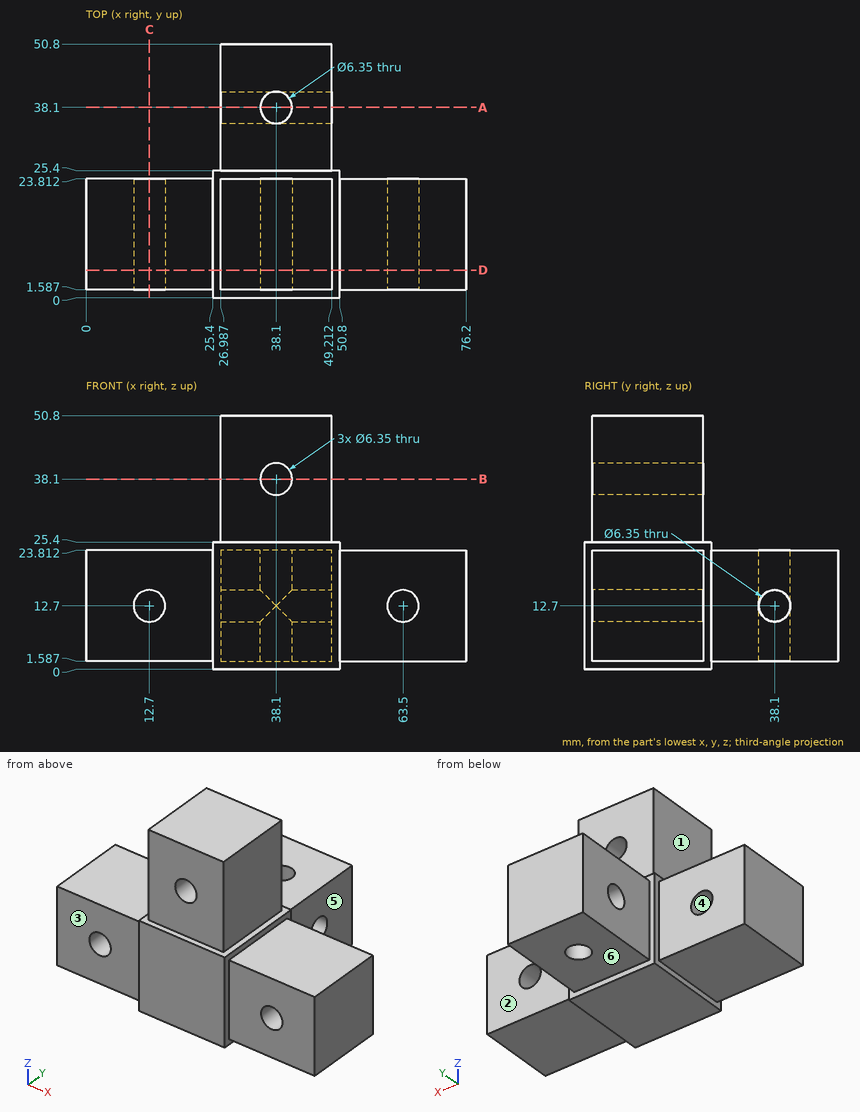
For this review, use the dimensioned drawing (mm, ordinates from the lowest corner) and the shaded views. A direction names the side the tool comes from. Round coordinates to 2 decimals unless told otherwise and drop trailing zeros. Order: outer loops, then holes, each group sorted by start corner. A loop starts at its lowest first (then second) coordinate and runs counter-clockwise, first axis right, second up. Notation, with made-up numbers: M 46.5,58 L 71.5,58 A20 cw 71.5,68 Z; hole C -28,55 d7. An arc over 180 degrees is marked long. Use a Markdown table: item, result.
1) Consider section A-A (y = 38.1). Write out the cut boundary in (x, z) (1 decimal).
Report:
| item | result |
|---|---|
| outline | M 27,1.6 L 34.9,1.6 L 34.9,9.5 L 27,9.5 Z; M 27,15.9 L 34.9,15.9 L 34.9,23.8 L 27,23.8 Z; M 41.3,1.6 L 49.2,1.6 L 49.2,9.5 L 41.3,9.5 Z; M 41.3,15.9 L 49.2,15.9 L 49.2,23.8 L 41.3,23.8 Z |
2) Wall thickness on line 1 along X through (y, z) = (16, 12.7) (1 decimal); line 2 along Y through (x, z) = (40.5, 13); line 3 along Z through (x, y) = (31, 38.1) (1 decimal): over which ranges is each line inside the solid? List them lowest first. Write a range as [from, to].
Report:
| item | result |
|---|---|
| line 1 | [0, 9.5], [15.9, 60.3], [66.7, 76.2] |
| line 2 | [0, 34.94], [41.26, 50.8] |
| line 3 | [1.6, 9.5], [15.9, 23.8] |
3) Consider section C-C (x = 12.7). Write out the cut boundary in (y, z) (1 decimal), then the cut area to 3 significant figures.
Report:
| item | result |
|---|---|
| outline | M 1.6,1.6 L 23.8,1.6 L 23.8,9.5 L 1.6,9.5 Z; M 1.6,15.9 L 23.8,15.9 L 23.8,23.8 L 1.6,23.8 Z |
| area | 353 mm^2 |
4) Consider section D-D (y = 5.5). Give the number of separate pieces and of enclosed holes in the cut face, then the cut area to 3 significant figures.
Report:
| item | result |
|---|---|
| separate pieces | 1 |
| enclosed holes | 3 |
| area | 2,240 mm^2 |
5) Consider section B-B (z = 38.1). Write out the cut boundary in (x, y) (1 decimal).
Report:
| item | result |
|---|---|
| outline | M 27,1.6 L 34.9,1.6 L 34.9,23.8 L 27,23.8 Z; M 41.3,1.6 L 49.2,1.6 L 49.2,23.8 L 41.3,23.8 Z |
6) Tool access review of the marked faces 1, 2 and 3: name each direction out of +Z, -Z, +X, -X, +Y, -Y from which nothing blocks a thin tool from reaching the whole face with its end or side.
Report:
| item | result |
|---|---|
| face 1 | +Z, -X, +Y, -Y |
| face 2 | +Z, -Z, +X, +Y |
| face 3 | +Z, -Z, -X, -Y |
7) Draft analysis for pull direction X (two halves, no side actions). For the marked faces 4, 5 and 6, state which applies: released by +X, released by -X, zero draft, split by the parting line, or undercut.
Report:
| item | result |
|---|---|
| face 4 | undercut |
| face 5 | released by +X |
| face 6 | zero draft |
8) Insertion check: pin 1 (18 mm diameter, centred on x = 66.5, z = 16, fed in from +Y); pin 2 (6.5 mm diameter, centred on y = 18, z = 43, fed in from -X); pin 3 (1.5 mm diameter, centred on x = 65.5, y = 20, fed in from -Z). Each pin has a flat end and moves straight along its axis. Give the tip position at first contact, or say it passes through.
Report:
| item | result |
|---|---|
| pin 1 | y = 23.81 |
| pin 2 | x = 26.99 |
| pin 3 | z = 1.59 |
